Check sheet for the modelled part. Datum: model origin and axes. Units: mm. A direction names the side the tool comes from. Coordinates: 2 decimals unless noted, no trailing zeros. Loops run counter-clockwise (first coordinate to the right, second up) from the corner with the lowest first, then second, coordinate; pieces in that order, holes last. Notation, with made-up numbers: (32, 38) - (81, 38) arc R17 cw to (81, 68) - close; hole circle Ø2 at (85.25, 63.5). An arc over 180 degrees is marked (long way). Write each question's results on one line, items separated by ' | '. Start each with the question number.
1. Cross-section at A-A (z = 30). Give the number of separate pieces and of enclosed holes in the cut face, and give its area (3 significant figures).
2. Draft check along X on faces 1 (the face through (33.6, 6, 30.9)), 2 (the face through (-32, 3, 31)), 3 (the face through (0, 1, 55)). Enter one of: released by +X, released by -X, zero draft, split by the parting line, or undercut.
3. Cross-section at D-D (x = -7). Record the cut outline in (y, z).
4. Cross-section at B-B (x = -35). Record the cut outline in (y, z), and give its area (3 significant figures).
5. Tool access check on faces 4 (the face through (33, 8, 31)), 5 (the face through (-12.5, 1, 32)), 6 (the face through (-13, 2, 31)), 7 (the face through (14, 0, 37)), 8 (the face through (-36.4, 6, 30.9)). Record the directions out of +Z, -Z, +X, -X, +Y, -Y that give a thin tool (end or side, any length) a straight path to the whole face; none if there is none.
6. Gauge pin test, flat ends, axial feed: P1, Ø5, axis at x = 22.5, z = 50.5, coming from the +Y side; P2, Ø1.5, axis at y = 3.5, z = 49, coming from the -X side; P3, Ø4, axis at x = 35, z = 10, coming from the -Y side; P4, Ø2.5, axis at x = 35, z = 50, coming from the +Y side. Record the tip position at first contact, or that the pin passes through.
7. Thickness scan on line 1 (Z direction, x = -15, y = 0.4); line 2 (Z direction, x = -35, y = 6.4); line 3 (X direction, y = 1.4, z = 13). Record the ranges inside material, lowest first. Write a range as [from, to].
8. Cross-section at C-C (z = 13). Record the cut outline in (x, y), and give its area (3 significant figures).
```python
from build123d import *

# Parameters (mm, degrees)
BOSS_EXTRUDE1_DEPTH            = 50
BOSS_EXTRUDE1_2_DEPTH          = 50
SKETCH4_W                      = 1.5
SKETCH4_H                      = 2
F_3_0MM_DOWEL_HOLE1_AT_2_COUNT = 2
F_3_0MM_DOWEL_HOLE1_AT_2_PITCH = 17
F_3_0MM_DOWEL_HOLE1_AT_3_COUNT = 2
F_3_0MM_DOWEL_HOLE1_AT_3_PITCH = 34
F_3_0MM_DOWEL_HOLE1_AT_4_COUNT = 2
F_3_0MM_DOWEL_HOLE1_AT_4_PITCH = 45.343136195
F_3_0MM_DOWEL_HOLE1_AT_5_COUNT = 2
F_3_0MM_DOWEL_HOLE1_AT_5_PITCH = 34.481879299
F_3_0MM_DOWEL_HOLE1_AT_6_COUNT = 2
F_3_0MM_DOWEL_HOLE1_AT_6_PITCH = 30
SKETCH7_W                      = 1.5
SKETCH7_H                      = 8
F_3_0MM_DOWEL_HOLE2_AT_2_COUNT = 2
F_3_0MM_DOWEL_HOLE2_AT_2_PITCH = 10
F_3_0MM_DOWEL_HOLE2_AT_3_COUNT = 2
F_3_0MM_DOWEL_HOLE2_AT_3_PITCH = 10
F_3_0MM_DOWEL_HOLE2_AT_4_COUNT = 2
F_3_0MM_DOWEL_HOLE2_AT_4_PITCH = 20
SKETCH9_W                      = 25
SKETCH9_H                      = 9
BOSS_EXTRUDE3_DEPTH            = 2
MIRROR1_COPY_1_SKETCH_W        = 1.5
MIRROR1_COPY_1_SKETCH_H        = 8
MIRROR1_COPY_2_SKETCH_W        = 1.5
MIRROR1_COPY_2_SKETCH_H        = 8
MIRROR1_COPY_3_SKETCH_W        = 1.5
MIRROR1_COPY_3_SKETCH_H        = 8
SKETCH10_W                     = 76
SKETCH10_H                     = 4
CUT_EXTRUDE1_DEPTH             = 10
BOSS_EXTRUDE4_DEPTH            = 8.5
SKETCH13_W                     = 25
SKETCH13_H                     = 5
CUT_EXTRUDE2_DEPTH             = 8.5
F_3_0MM_DOWEL_HOLE3_D          = 3


with BuildPart() as part:
    # Sketch1 → Boss-Extrude1 (new body)
    with BuildSketch(Plane.XY):
        Polygon((12.5, 0), (12.5, 2), (30, 2), (30, 8), (38, 8), (38, 6), (32, 6), (32, 0), align=None)
    extrude(amount=BOSS_EXTRUDE1_DEPTH)


with BuildPart() as body_2:
    # Sketch1 → Boss-Extrude1 2 (new body)
    with BuildSketch(Plane.XY):
        Polygon((-12.5, 2), (-30, 2), (-30, 8), (-38, 8), (-38, 6), (-32, 6), (-32, 0), (-12.5, 0), align=None)
    extrude(amount=BOSS_EXTRUDE1_2_DEPTH)

    # Sketch4 → Ø3.0mm Dowel Hole1 (revolve, cut)
    with BuildSketch(Plane(origin=(-15, 2, 47), x_dir=(0, 0, 1), z_dir=(1, 0, 0))):
        with Locations((0.75, 1)):
            Rectangle(SKETCH4_W, SKETCH4_H)
    f_3_0mm_dowel_hole1 = revolve(axis=Axis((-15, 8.35, 47), (0, -1, 0)), mode=Mode.SUBTRACT)

    # Ø3.0mm Dowel Hole1 at 2: Ø3.0mm Dowel Hole1 ×2
    with Locations(*[(0, 0, -i * F_3_0MM_DOWEL_HOLE1_AT_2_PITCH) for i in range(1, F_3_0MM_DOWEL_HOLE1_AT_2_COUNT)]):
        add(f_3_0mm_dowel_hole1, mode=Mode.SUBTRACT)

    # Ø3.0mm Dowel Hole1 at 3: Ø3.0mm Dowel Hole1 ×2
    with Locations(*[(0, 0, -i * F_3_0MM_DOWEL_HOLE1_AT_3_PITCH) for i in range(1, F_3_0MM_DOWEL_HOLE1_AT_3_COUNT)]):
        add(f_3_0mm_dowel_hole1, mode=Mode.SUBTRACT)

    # Sketch7 → Ø3.0mm Dowel Hole2 (revolve, cut)
    with BuildSketch(Plane(origin=(-35, 8, 20), x_dir=(0, 0, 1), z_dir=(1, 0, 0))):
        with Locations((0.75, 4)):
            Rectangle(SKETCH7_W, SKETCH7_H)
    f_3_0mm_dowel_hole2 = revolve(axis=Axis((-35, 14.35, 20), (0, -1, 0)), mode=Mode.SUBTRACT)

    # Ø3.0mm Dowel Hole2 at 2: Ø3.0mm Dowel Hole2 ×2
    with Locations(*[(0, 0, -i * F_3_0MM_DOWEL_HOLE2_AT_2_PITCH) for i in range(1, F_3_0MM_DOWEL_HOLE2_AT_2_COUNT)]):
        add(f_3_0mm_dowel_hole2, mode=Mode.SUBTRACT)

    # Ø3.0mm Dowel Hole2 at 3: Ø3.0mm Dowel Hole2 ×2
    with Locations(*[(0, 0, i * F_3_0MM_DOWEL_HOLE2_AT_3_PITCH) for i in range(1, F_3_0MM_DOWEL_HOLE2_AT_3_COUNT)]):
        add(f_3_0mm_dowel_hole2, mode=Mode.SUBTRACT)

    # Ø3.0mm Dowel Hole2 at 4: Ø3.0mm Dowel Hole2 ×2
    with Locations(*[(0, 0, i * F_3_0MM_DOWEL_HOLE2_AT_4_PITCH) for i in range(1, F_3_0MM_DOWEL_HOLE2_AT_4_COUNT)]):
        add(f_3_0mm_dowel_hole2, mode=Mode.SUBTRACT)


with BuildPart() as part_1:
    add(part.part)

    # Ø3.0mm Dowel Hole1 at 4: Ø3.0mm Dowel Hole1 ×2
    with Locations(*[Vector(0.661621637, 0, -0.749837855) * (i * F_3_0MM_DOWEL_HOLE1_AT_4_PITCH) for i in range(1, F_3_0MM_DOWEL_HOLE1_AT_4_COUNT)]):
        add(f_3_0mm_dowel_hole1, mode=Mode.SUBTRACT)

    # Ø3.0mm Dowel Hole1 at 5: Ø3.0mm Dowel Hole1 ×2
    with Locations(*[Vector(0.870022186, 0, -0.493012572) * (i * F_3_0MM_DOWEL_HOLE1_AT_5_PITCH) for i in range(1, F_3_0MM_DOWEL_HOLE1_AT_5_COUNT)]):
        add(f_3_0mm_dowel_hole1, mode=Mode.SUBTRACT)

    # Ø3.0mm Dowel Hole1 at 6: Ø3.0mm Dowel Hole1 ×2
    with Locations(*[(i * F_3_0MM_DOWEL_HOLE1_AT_6_PITCH, 0, 0) for i in range(1, F_3_0MM_DOWEL_HOLE1_AT_6_COUNT)]):
        add(f_3_0mm_dowel_hole1, mode=Mode.SUBTRACT)

    add(body_2.part)  # Boss-Extrude3 merges body 2
    # Sketch9 → Boss-Extrude3 (add)
    with BuildSketch(Plane(origin=(0, 2, 0), x_dir=(1, 0, 0), z_dir=(0, 1, 0))):
        with Locations((0, -4.5)):
            Rectangle(SKETCH9_W, SKETCH9_H)
    extrude(amount=-BOSS_EXTRUDE3_DEPTH)

    # Mirror1: Ø3.0mm Dowel Hole2 across plane
    add(f_3_0mm_dowel_hole2.mirror(Plane(origin=(0, 0, 0), x_dir=(0, 0, 1), z_dir=(1, 0, 0))), mode=Mode.SUBTRACT)

    # Mirror1 copy 1 sketch → Mirror1 copy 1 (revolve, cut)
    with BuildSketch(Plane(origin=(35, 8, 10), x_dir=(0, 0, 1), z_dir=(-1, 0, 0))):
        with Locations((0.75, -4)):
            Rectangle(MIRROR1_COPY_1_SKETCH_W, MIRROR1_COPY_1_SKETCH_H)
    revolve(axis=Axis((35, 14.35, 10), (0, 1, 0)), mode=Mode.SUBTRACT)

    # Mirror1 copy 2 sketch → Mirror1 copy 2 (revolve, cut)
    with BuildSketch(Plane(origin=(35, 8, 30), x_dir=(0, 0, 1), z_dir=(-1, 0, 0))):
        with Locations((0.75, -4)):
            Rectangle(MIRROR1_COPY_2_SKETCH_W, MIRROR1_COPY_2_SKETCH_H)
    revolve(axis=Axis((35, 14.35, 30), (0, 1, 0)), mode=Mode.SUBTRACT)

    # Mirror1 copy 3 sketch → Mirror1 copy 3 (revolve, cut)
    with BuildSketch(Plane(origin=(35, 8, 40), x_dir=(0, 0, 1), z_dir=(-1, 0, 0))):
        with Locations((0.75, -4)):
            Rectangle(MIRROR1_COPY_3_SKETCH_W, MIRROR1_COPY_3_SKETCH_H)
    revolve(axis=Axis((35, 14.35, 40), (0, 1, 0)), mode=Mode.SUBTRACT)

    # Sketch10 → Cut-Extrude1 (cut)
    with BuildSketch(Plane(origin=(0, 8, 0), x_dir=(1, 0, 0), z_dir=(0, 1, 0))):
        with Locations((0, -2)):
            Rectangle(SKETCH10_W, SKETCH10_H)
    extrude(amount=-CUT_EXTRUDE1_DEPTH, mode=Mode.SUBTRACT)

    # Sketch12 → Boss-Extrude4 (add)
    with BuildSketch(Plane.XY.offset(50)):
        Polygon((-32, 0), (32, 0), (32, 6), (38, 6), (38, 8), (30, 8), (30, 2), (-30, 2), (-30, 8), (-38, 8), (-38, 6), (-32, 6), align=None)
    extrude(amount=BOSS_EXTRUDE4_DEPTH)

    # Sketch13 → Cut-Extrude2 (cut)
    with BuildSketch(Plane(origin=(0, 2, 0), x_dir=(1, 0, 0), z_dir=(0, 1, 0))):
        with Locations((0, -52.5)):
            Rectangle(SKETCH13_W, SKETCH13_H)
    extrude(amount=-CUT_EXTRUDE2_DEPTH, mode=Mode.SUBTRACT)

    # Ø3.0mm Dowel Hole3 (through all)
    with Locations(Plane(origin=(0, 8, 0), x_dir=(1, 0, 0), z_dir=(0, 1, 0))):
        with Locations((35, -50), (-35, -50)):
            Hole(F_3_0MM_DOWEL_HOLE3_D / 2)


solid = part_1.part
```
Established:
1) separate pieces: 6 | enclosed holes: 0 | area: 102 mm^2
2) face 1: zero draft | face 2: released by -X | face 3: undercut
3) outline: (0, 4) - (2, 4) - (2, 9) - (0, 9) - close; (0, 55) - (2, 55) - (2, 58.5) - (0, 58.5) - close
4) outline: (6, 4) - (8, 4) - (8, 8.5) - (6, 8.5) - close; (6, 11.5) - (8, 11.5) - (8, 18.5) - (6, 18.5) - close; (6, 21.5) - (8, 21.5) - (8, 28.5) - (6, 28.5) - close; (6, 31.5) - (8, 31.5) - (8, 38.5) - (6, 38.5) - close; (6, 41.5) - (8, 41.5) - (8, 48.5) - (6, 48.5) - close; (6, 51.5) - (8, 51.5) - (8, 58.5) - (6, 58.5) - close | area: 79.0 mm^2
5) face 4: +Z, -Z, +X, -X, +Y | face 5: +Y, -Y | face 6: +Z, -Z, +Y | face 7: +Z, -Z, +X, -X, -Y | face 8: +Z, -Z, -X, -Y
6) P1: y = 2 | P2: x = -32 | P3: y = 6 | P4: through
7) line 1: [4, 11.5], [14.5, 28.5], [31.5, 45.5], [48.5, 58.5] | line 2: [4, 8.5], [11.5, 18.5], [21.5, 28.5], [31.5, 38.5], [41.5, 48.5], [51.5, 58.5] | line 3: [-32, -16.5], [-13.5, -12.5], [12.5, 13.5], [16.5, 32]
8) outline: (-38, 6) - (-32, 6) - (-32, 0) - (-16.5, 0) - (-16.5, 2) - (-30, 2) - (-30, 8) - (-38, 8) - close; (-13.5, 0) - (-12.5, 0) - (-12.5, 2) - (-13.5, 2) - close; (12.5, 0) - (13.5, 0) - (13.5, 2) - (12.5, 2) - close; (16.5, 0) - (32, 0) - (32, 6) - (38, 6) - (38, 8) - (30, 8) - (30, 2) - (16.5, 2) - close | area: 114 mm^2
